Work out the finished part from the listing and answer in its coordinate system (mm). A direction names the side the tool comes from. Round coordinates to 2 decimals unless told otherwise and drop trailing zeros. Write each loop counter-clockwise with the first axis right and the second up, starting at its lowest first coordinate (ties: lowest second). Pieces come first, ordered by that corner, then holes. Notation, with made-up numbers: M 26.25,64.5 L 39.25,64.5 A20 ccw 39.25,102.5 Z; hole C 60,76.5 d6. An arc over 180 degrees is marked long. Answer in a Markdown table with one row per item.
```python
from build123d import *

# Parameters (mm, degrees)
SKETCH2_W           = 41.77
SKETCH2_H           = 60
BOSS_EXTRUDE1_DEPTH = 28.08
SKETCH6_W           = 15
SKETCH6_H           = 10
BOSS_EXTRUDE4_DEPTH = 90
SKETCH7_W           = 6.4
SKETCH7_H           = 12.4
CUT_EXTRUDE1_DEPTH  = 135.955250454
SKETCH8_W           = 51
SKETCH8_H           = 18.08
BOSS_EXTRUDE5_DEPTH = 50
SKETCH9_W           = 33
SKETCH9_H           = 13.08
CUT_EXTRUDE2_DEPTH  = 32
SKETCH10_W          = 35.77
SKETCH10_H          = 54
CUT_EXTRUDE3_DEPTH  = 25.08
SKETCH11_W          = 50
SKETCH11_H          = 9
CUT_EXTRUDE4_DEPTH  = 15.08
SKETCH13_R          = 10.4
CUT_EXTRUDE5_DEPTH  = 10
CHAMFER1_SIZE       = 1


with BuildPart() as part:
    # Sketch2 → Boss-Extrude1 (new body)
    with BuildSketch(Plane(origin=(0, 0, 0), x_dir=(1, 0, 0), z_dir=(0, 1, 0))):
        with Locations((-5, 0)):
            Rectangle(SKETCH2_W, SKETCH2_H)
    extrude(amount=BOSS_EXTRUDE1_DEPTH)

    # Sketch6 → Boss-Extrude4 (add)
    with BuildSketch(Plane(origin=(0, 28.08, 0), x_dir=(1, 0, 0), z_dir=(0, 1, 0))):
        with Locations((0, -25)):
            Rectangle(SKETCH6_W, SKETCH6_H)
        with Locations((0, 25)):
            Rectangle(SKETCH6_W, SKETCH6_H)
    extrude(amount=BOSS_EXTRUDE4_DEPTH)

    # Sketch7 → Cut-Extrude1 (cut, through all)
    with BuildSketch(Plane(origin=(0, 0, -30), x_dir=(-1, 0, 0), z_dir=(0, 0, -1))):
        with Locations((0, 111.88)):
            Rectangle(SKETCH7_W, SKETCH7_H)
    extrude(amount=-CUT_EXTRUDE1_DEPTH, mode=Mode.SUBTRACT)

    # Sketch8 → Boss-Extrude5 (add)
    with BuildSketch(Plane(origin=(15.885, 0, 0), x_dir=(0, 0, -1), z_dir=(1, 0, 0))):
        with Locations((25.5, 9.04)):
            Rectangle(SKETCH8_W, SKETCH8_H)
    extrude(amount=BOSS_EXTRUDE5_DEPTH)

    # Sketch9 → Cut-Extrude2 (cut)
    with BuildSketch(Plane(origin=(55.885, 0, 0), x_dir=(0, 0, -1), z_dir=(1, 0, 0))):
        with Locations((29.5, 11.54)):
            Rectangle(SKETCH9_W, SKETCH9_H)
    extrude(amount=-CUT_EXTRUDE2_DEPTH, mode=Mode.SUBTRACT)

    # Sketch10 → Cut-Extrude3 (cut)
    with BuildSketch(Plane.XZ):
        with Locations((-5, 0)):
            Rectangle(SKETCH10_W, SKETCH10_H)
    extrude(amount=-CUT_EXTRUDE3_DEPTH, mode=Mode.SUBTRACT)

    # Sketch11 → Cut-Extrude4 (cut)
    with BuildSketch(Plane.XZ):
        with Locations((37.885, -7.5)):
            Rectangle(SKETCH11_W, SKETCH11_H)
    extrude(amount=-CUT_EXTRUDE4_DEPTH, mode=Mode.SUBTRACT)

    # Sketch13 → Cut-Extrude5 (cut)
    with BuildSketch(Plane(origin=(0, 5, 0), x_dir=(1, 0, 0), z_dir=(0, 1, 0))):
        with Locations(Location((39.885, 28.5, 0), (0, 0, 270))):
            Circle(SKETCH13_R)
    extrude(amount=-CUT_EXTRUDE5_DEPTH, mode=Mode.SUBTRACT)

    # Chamfer1
    chamfer1_edges = [part.edges().sort_by_distance(p)[0] for p in [
        (39.885, 5, -38.9),
    ]]
    chamfer(chamfer1_edges, length=CHAMFER1_SIZE)


solid = part.part
```
1. Determine the mould class of faces 5 (the flat face through (38, 7, -12)), 6 (the flat face through (15.885, 9, -40)), 7 (the flat face through (-5, 118.08, 25)) for opening direction X: released by +X, released by -X, zero draft, split by the parting line, or undercut.
Calculated:
| item | result |
|---|---|
| face 5 | undercut |
| face 6 | released by -X |
| face 7 | zero draft |
2. Consider line 1 along X through (y, z) = (1, -28) (3 decimals); line 2 along Z through (x, y) = (5.5, 50.5); line 3 along X through (y, z) = (13.5, -27.5) (3 decimals). Determine where each line is inside the solid, lowest interval first. Write a range as from..to.
Calculated:
| item | result |
|---|---|
| line 1 | x = -25.885..29.497, 50.273..65.885 |
| line 2 | z = -30..-20, 20..30 |
| line 3 | x = -25.885..23.885, 55.885..65.885 |
3. The part is cut by section C-C (y = 12.5). Determine the outline of the cut face in (x, z) (3 decimals).
Calculated:
| item | result |
|---|---|
| outline | M -25.885,-30 L 15.885,-30 L 15.885,-51 L 65.885,-51 L 65.885,0 L 15.885,0 L 15.885,30 L -25.885,30 Z; hole M -22.885,-27 L 12.885,-27 L 12.885,-12 L 62.885,-12 L 62.885,-3 L 12.885,-3 L 12.885,27 L -22.885,27 Z; hole M 23.885,-46 L 55.885,-46 L 55.885,-13 L 23.885,-13 Z |
4. The part is cut by section B-B (y = 39). Determine the outline of the cut face in (x, z).
Calculated:
| item | result |
|---|---|
| outline | M -7.5,-30 L 7.5,-30 L 7.5,-20 L -7.5,-20 Z; M -7.5,20 L 7.5,20 L 7.5,30 L -7.5,30 Z |
5. Given pin 1 (3 mm diameter, centred on y = 77.5, z = -24.5, fed in from -X); pin 2 (11 mm diameter, centred on y = 66, z = -26, fed in from +X); pin 3 (4 mm diameter, centred on y = 8.5, z = -35.5, fed in from -X) (3 decimals); pin 4 (7 mm diameter, centred on x = -0.5, z = 25.5, fed in from +Y), each flat-ended and moving along its own axis, determine where each tip first touches the part or whether it passes through.
Calculated:
| item | result |
|---|---|
| pin 1 | stops at x = -7.5 |
| pin 2 | stops at x = 7.5 |
| pin 3 | stops at x = 15.885 |
| pin 4 | stops at y = 118.08 |
6. A tool of negligible diameter and unlimited length cuts with its end or side. For faces 1 (the flat face through (0, 72, -20)), 2 (the flat face through (41, 18.08, -8)), 3 (the flat face through (-3.2, 112, 25)), 4 (the flat face through (38, 15.08, -7)), from which of +Z, -Z, +X, -X, +Y, -Y can it reach the whole face along a straight path? Write none if from no direction.
Calculated:
| item | result |
|---|---|
| face 1 | +X, -X, +Y |
| face 2 | +Z, -Z, +X, +Y |
| face 3 | +Z, -Z, +Y |
| face 4 | -Y |
7. The part is cut by section D-D (x = -1). Determine the outline of the cut face in (y, z), plus the area to 3 significant figures.
Calculated:
| item | result |
|---|---|
| outline | M 0,-30 L 105.68,-30 L 105.68,-20 L 28.08,-20 L 28.08,20 L 105.68,20 L 105.68,30 L 0,30 L 0,27 L 25.08,27 L 25.08,-27 L 0,-27 Z |
| area | 1,880 mm² |
8. The part is cut by section A-A (z = -28.5). Determine the outline of the cut face in (x, y) (3 decimals), plus the area to 3 significant figures.
Calculated:
| item | result |
|---|---|
| outline | M -25.885,0 L 29.485,0 L 29.485,4 L 28.485,5 L 23.885,5 L 23.885,18.08 L 15.885,18.08 L 15.885,28.08 L 7.5,28.08 L 7.5,118.08 L 3.2,118.08 L 3.2,105.68 L -3.2,105.68 L -3.2,118.08 L -7.5,118.08 L -7.5,28.08 L -25.885,28.08 Z; M 50.285,0 L 65.885,0 L 65.885,18.08 L 55.885,18.08 L 55.885,5 L 51.285,5 L 50.285,4 Z |
| area | 2,820 mm² |
